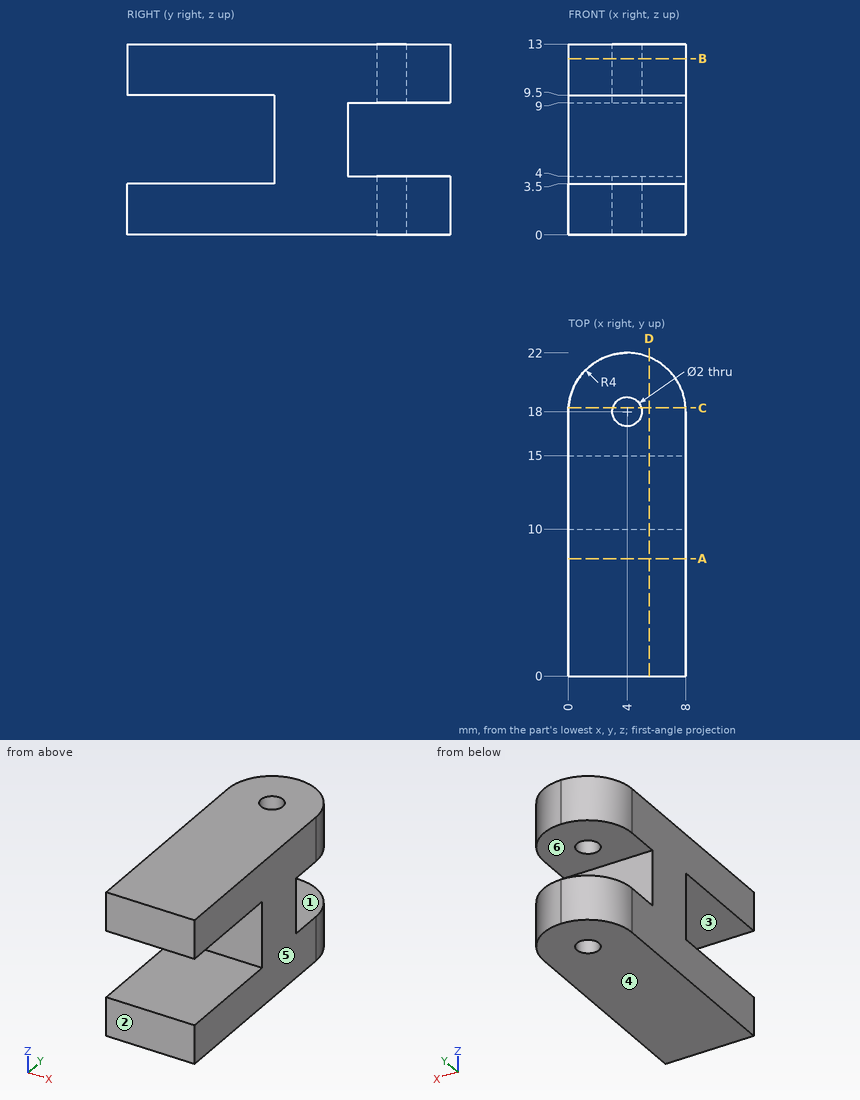
Print and shaded views of the part. All mm, measured from the part's lowest x, y and z. A direction names the side the tool comes from. Coordinates: 2 decimals unless noted, no trailing zeros. Loops run counter-clockwise (first coordinate to the right, second up) from the corner with the lowest first, then second, coordinate; pieces in that order, holes last. Notation, with made-up numbers: (86, -8.5) -> (90, -8.5) arc R21 ccw to (90, -4.5) -> close; hole circle Ø9 at (33, 72.25). An arc over 180 degrees is marked (long way). Use one line per item in the form item = value. Start each with the question number.
(1) Cut at B-B on z = 12. Give the cut face in (x, y), and give its area (3 significant figures).
(2) Cut at A-A on y = 8. Give the cut face in (x, z), and give its area (3 significant figures).
(3) Pull direction Z, two halves, no side cores. Call the marked faces 4, 5 and 6: pulls with the +Z half, pulls with the -Z half, needs draft (parallel to the pull), parting line crosses it, or undercut.
(4) Probe probe 1 along Z at (x, y) = (5.75, 1.75); probe 2 along Z at (x, y) = (7.75, 15.5); probe 3 along Y at (x, z) = (4, 0.95). List the from-to ranges inside material, lowest first. Write a range as from..to.
(5) Tool access for the marked faces 1, 2 and 3: list every direction of +Z, -Z, +X, -X, +Y, -Y with a clear straight run to the whole face (end or side of a thin tool).
(6) Cut at C-C on y = 18.25. Give the cut face in (x, z).
(7) Flat gauge pins, fed straight in: pin 1 (1.8 mm diameter, centred on x = 5.5, z = 6.5, fed in from -Y); pin 2 (1.6 mm diameter, centred on x = 4, y = 18, fed in from +Z); pin 3 (1.5 mm diameter, centred on x = 4.5, z = 6, fed in from +Y). Where does each tip first touch, or does it go through?
(8) Cut at D-D on x = 5.5. Give the cut face in (y, z), and give its area (3 significant figures).
Values:
q1.outline = (0, 0) -> (8, 0) -> (8, 18) arc R4 ccw to (0, 18) -> close; hole circle Ø2 at (4, 18)
q1.area = 166 mm2
q2.outline = (0, 0) -> (8, 0) -> (8, 3.5) -> (0, 3.5) -> close; (0, 9.5) -> (8, 9.5) -> (8, 13) -> (0, 13) -> close
q2.area = 56.0 mm2
q3.face_4 = pulls with the -Z half
q3.face_5 = needs draft
q3.face_6 = undercut
q4.probe_1 = 0..3.5, 9.5..13
q4.probe_2 = 0..4, 9..13
q4.probe_3 = 0..17, 19..22
q5.face_1 = +X, -X, +Y
q5.face_2 = +Z, -Z, +X, -X, -Y
q5.face_3 = +X, -X, -Y
q6.outline = (0.01, 0) -> (3.03, 0) -> (3.03, 4) -> (0.01, 4) -> close; (0.01, 9) -> (3.03, 9) -> (3.03, 13) -> (0.01, 13) -> close; (4.97, 0) -> (7.99, 0) -> (7.99, 4) -> (4.97, 4) -> close; (4.97, 9) -> (7.99, 9) -> (7.99, 13) -> (4.97, 13) -> close
q7.pin_1 = 10
q7.pin_2 = through
q7.pin_3 = 15
q8.outline = (0, 0) -> (21.71, 0) -> (21.71, 4) -> (15, 4) -> (15, 9) -> (21.71, 9) -> (21.71, 13) -> (0, 13) -> (0, 9.5) -> (10, 9.5) -> (10, 3.5) -> (0, 3.5) -> close
q8.area = 189 mm2
